from build123d import *

# Parameters (mm, degrees)
F0_W      = 127
F0_H      = 76.2
F1_DEPTH  = 25.4
F2_R      = 5.08
F4_W      = 8
F4_H      = 16.4
F5_DEPTH  = 16
F6_W      = 8
F6_H      = 16.4
F7_DEPTH  = 16
F8_R      = 8.490397
F9_DEPTH  = 1
F10_W     = 8.591677
F10_H     = 4.027348
F11_DEPTH = 16


with BuildPart() as f1:
    # F0 (on Front) → F1 (new body)
    with BuildSketch(Plane.XZ):
        Rectangle(F0_W, F0_H)
    extrude(amount=F1_DEPTH)

    # F2
    f2_edges = [f1.edges().sort_by_distance(p)[0] for p in [
        (0, -25.4, 38.1),
        (0, 0, 38.1),
        (0, 0, -38.1),
        (0, -25.4, -38.1),
    ]]
    fillet(f2_edges, radius=F2_R)

    # F4 (on face) → F5 (cut)
    with BuildSketch(Plane.YZ.offset(63.5)):
        with Locations((-17.896974, 23.987068)):
            Rectangle(F4_W, F4_H)
    extrude(amount=-F5_DEPTH, mode=Mode.SUBTRACT)

    # F6 (on face) → F7 (cut)
    with BuildSketch(Plane.YZ.offset(63.5)):
        with Locations((-7.068553, 24.406013)):
            Rectangle(F6_W, F6_H)
    extrude(amount=-F7_DEPTH, mode=Mode.SUBTRACT)

    # F8 (on face) → F9 (join)
    with BuildSketch(Plane.YZ.offset(63.5)):
        with Locations((-13.021762, -7.383473)):
            Circle(F8_R)
    extrude(amount=F9_DEPTH)

    # F10 (on face) → F11 (cut)
    with BuildSketch(Plane.YZ.offset(63.5)):
        with Locations((-12.484782, -23.627115)):
            Rectangle(F10_W, F10_H)
    extrude(amount=-F11_DEPTH, mode=Mode.SUBTRACT)


solid = f1.part
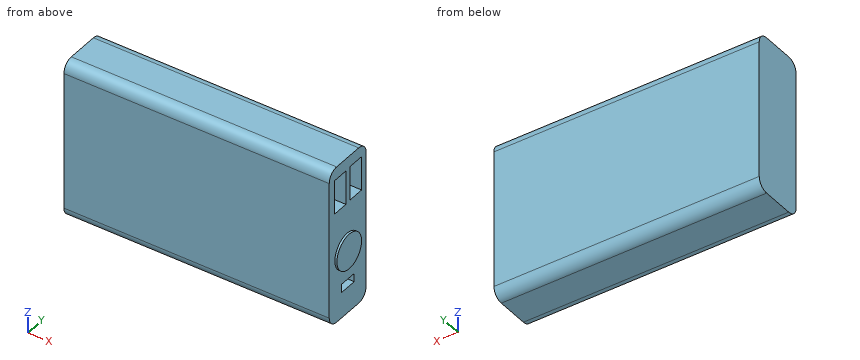
Read the model definition and answer for the solid it produces. Units are mm, in the model's axes. Give positions to 0.01 mm unless a question says otherwise; leave off trailing zeros. Write each loop counter-clockwise with the first axis right and the second up, starting at its lowest first coordinate (ties: lowest second). Pieces come first, ordered by that corner, then holes. Notation, with made-up numbers: (25.5, 72.25) - (52.5, 72.25) arc R10 cw to (52.5, 86.25) - close; hole circle Ø9 at (8, 43). An arc over 180 degrees is marked (long way). Return JSON: item names as keys, results as strings.
Q1. A cutting plane is placed at B-B, the plane y = -9.75. Determine the outline of the cut face in (x, z), and give its area (3 significant figures).
Reply:
{"outline": "(-63.5, -38.1) - (63.5, -38.1) - (63.5, -25.64) - (47.5, -25.64) - (47.5, -21.61) - (63.5, -21.61) - (63.5, -15.22) - (64.5, -15.22) - (64.5, 0.45) - (63.5, 0.45) - (63.5, 16.21) - (47.5, 16.21) - (47.5, 32.61) - (63.5, 32.61) - (63.5, 38.1) - (-63.5, 38.1) - close", "area": "9,370 mm²"}
Q2. A cutting plane is placed at C-C, the plane z = -24. Determine the outline of the cut face in (x, y).
Reply:
{"outline": "(-63.5, -25.4) - (63.5, -25.4) - (63.5, -16.78) - (47.5, -16.78) - (47.5, -8.19) - (63.5, -8.19) - (63.5, 0) - (-63.5, 0) - close"}
Q3. Consider line 1 along X through (y, z) = (-18.75, -25.5); line 2 along Z through (x, y) = (54, -6.5); line 3 along X through (y, z) = (-17.25, 30). Determine where each line is inside the solid, lowest interval first. Write a range as [from, to].
Reply:
{"line 1": "[-63.5, 63.5]", "line 2": "[-38.1, 16.21], [32.61, 38.1]", "line 3": "[-63.5, 47.5]"}
Q4. A cutting plane is placed at A-A, the plane z = 19. Determine the outline of the cut face in (x, y), and give its area (3 significant figures).
Reply:
{"outline": "(-63.5, -25.4) - (63.5, -25.4) - (63.5, -21.9) - (47.5, -21.9) - (47.5, -13.9) - (63.5, -13.9) - (63.5, -11.07) - (47.5, -11.07) - (47.5, -3.07) - (63.5, -3.07) - (63.5, 0) - (-63.5, 0) - close", "area": "2,970 mm²"}
Q5. Given P1, Ø4, axis at y = -20, z = 14, coming from the +X side; P2, Ø2.5, axis at y = -18.5, z = 26, coming from the +X side; P3, Ø2, axis at x = 15, y = -21.5, coming from the -Z side, each flat-ended and moving along its own axis, determine where each tip first touches the part or whether it passes through.
Reply:
{"P1": "x = 63.5", "P2": "x = 47.5", "P3": "z = -38.1"}
